Input: dimensioned drawing with shaded views. Units: mm. Origin: part minimum x, y, z. A direction names the side the tool comes from. Give positions to 0.01 mm unless a question says otherwise; leave off trailing zeros. Write each loop counter-clockwise with the first axis right and the second up, starting at its lowest first coordinate (ties: lowest second). Pieces come first, ordered by that corner, then holes. Notation, with made-up numbers: M 37,-15.75 L 75,-15.75 A14 ccw 75,9.25 Z; hole C 77,40.5 d2. An arc over 180 degrees is marked long. Use CSV: the item, a comma, the result in double quotes. Start each with the question number.
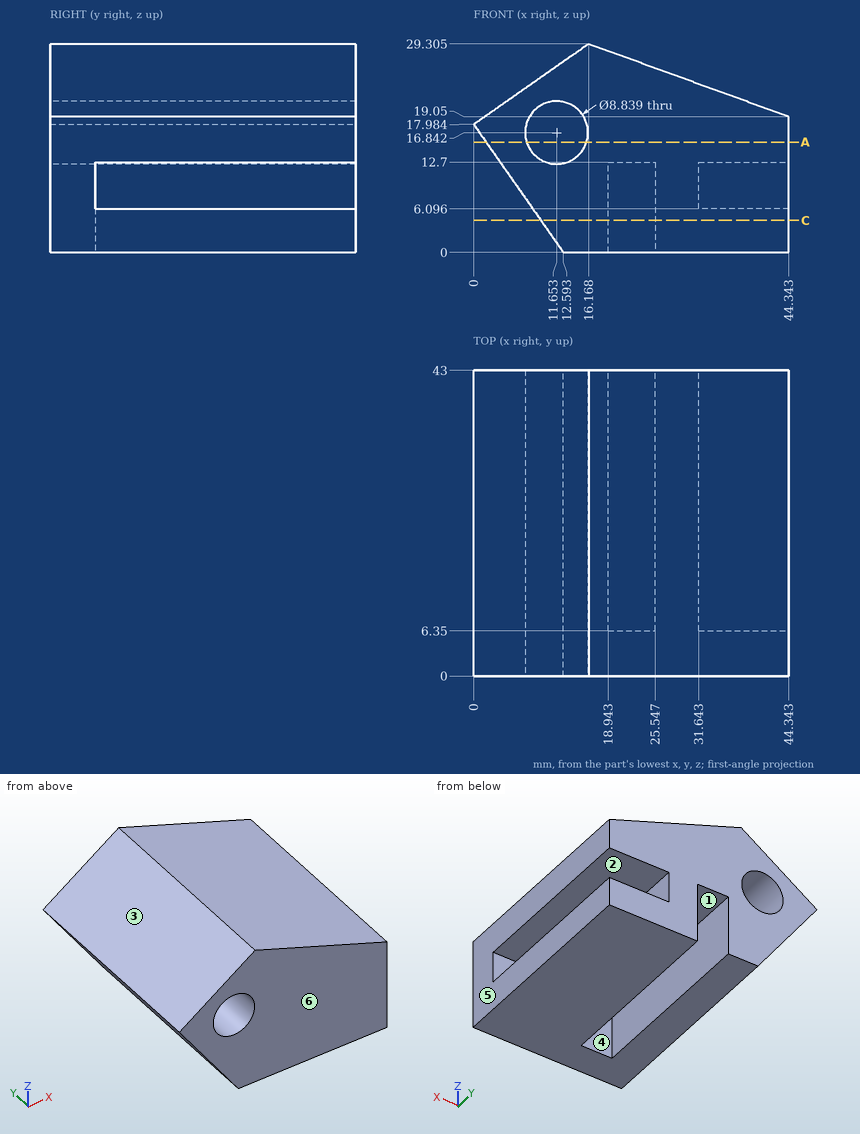
Item 1: Pull-direction query (X, two-part tool) for the marked faces 4, 5 and 6; classes: released by +X, released by -X, zero draft, split by the parting line, or undercut.
Item 2: Material intervals for probe 1 along Z at (x, y) = (26.5, 36) (1 decimal); probe 2 along X at (y, z) = (11, 5) (1 decimal); probe 3 along X at (y, z) = (25.5, 16.5) (1 decimal), sorted ascending.
Item 3: Contact query for flat-ended pins moving along their axis: pin 1 Ø1 at (x, y) = (29.5, 8) entering from +Z (1 decimal); pin 2 Ø2 at (x, z) = (36, 8.5) entering from +Y; pin 3 Ø1 at (x, y) = (34, 9) entering from +Z. Output: stop coordinate, or through.
Item 4: Set-up query: the marked faces 1, 2 and 3. Return all of +Z, -Z, +X, -X, +Y, -Y with unobstructed straight access to the full face (end or side cutting, diameter ignored); none if empty.
Item 5: Section A-A (z = 15.5). Return the cut outline in (x, y) (1 decimal).
Item 6: Section C-C (z = 4.5). Return the cut outline in (x, y).
Output values:
1,face 4,"undercut"
1,face 5,"released by +X"
1,face 6,"zero draft"
2,probe 1,"z = 0 to 25.5"
2,probe 2,"x = 9.1 to 18.9, 25.5 to 44.3"
2,probe 3,"x = 1 to 7.2, 16.1 to 44.3"
3,pin 1,"stops at z = 24.6"
3,pin 2,"stops at y = 6.35"
3,pin 3,"stops at z = 23"
4,face 1,"-Z, +Y"
4,face 2,"+X, +Y"
4,face 3,"+Z, -X, +Y, -Y"
5,outline,"M 1.7,0 L 7.4,0 L 7.4,43 L 1.7,43 Z; M 15.9,0 L 44.3,0 L 44.3,43 L 15.9,43 Z"
6,outline,"M 9.44,0 L 44.34,0 L 44.34,43 L 25.55,43 L 25.55,6.35 L 18.94,6.35 L 18.94,43 L 9.44,43 Z"
